from build123d import *

# Parameters (mm, degrees)
F0_W      = 12.7
F0_H      = 114.3
F1_DEPTH  = 12.7
F2_W      = 6.35
F2_H      = 12.7
F3_DEPTH  = 12.701
F4_R      = 2.794
F5_DEPTH  = 6.351
F6_R      = 4.7625
F7_DEPTH  = 5.08
F8_R      = 2.413
F9_DEPTH  = 9.525
F10_R     = 2.413
F11_DEPTH = 9.525


with BuildPart() as f1:
    # F0 (on Right) → F1 (new body)
    with BuildSketch(Plane.YZ):
        with Locations((-6.35, 0)):
            Rectangle(F0_W, F0_H)
    extrude(amount=F1_DEPTH)

    # F2 (on face) → F3 (cut, through all)
    with BuildSketch(Plane(origin=(0, 0, 0), x_dir=(-1, 0, 0), z_dir=(0, 1, 0))):
        with Locations((-3.175, 25.4)):
            Rectangle(F2_W, F2_H)
        with Locations((-3.175, -25.4)):
            Rectangle(F2_W, F2_H)
    extrude(amount=-F3_DEPTH, mode=Mode.SUBTRACT)

    # F4 (on face) → F5 (cut, through all)
    with BuildSketch(Plane(origin=(6.35, 0, 0), x_dir=(0, -1, 0), z_dir=(-1, 0, 0))):
        with Locations((6.35, 25.4)):
            Circle(F4_R)
        with Locations((6.35, -25.4)):
            Circle(F4_R)
    extrude(amount=-F5_DEPTH, mode=Mode.SUBTRACT)

    # F6 (on face) → F7 (cut)
    with BuildSketch(Plane.YZ.offset(12.7)):
        with Locations((-6.35, 25.4)):
            Circle(F6_R)
        with Locations((-6.35, -25.4)):
            Circle(F6_R)
    extrude(amount=-F7_DEPTH, mode=Mode.SUBTRACT)

    # F8 (on face) → F9 (cut)
    with BuildSketch(Plane.XY.offset(57.15)):
        with Locations((6.35, -6.35)):
            Circle(F8_R)
    extrude(amount=-F9_DEPTH, mode=Mode.SUBTRACT)

    # F10 (on face) → F11 (cut)
    with BuildSketch(Plane(origin=(0, 0, -57.15), x_dir=(1, 0, 0), z_dir=(0, 0, -1))):
        with Locations((6.35, 6.35)):
            Circle(F10_R)
    extrude(amount=-F11_DEPTH, mode=Mode.SUBTRACT)


solid = f1.part
Work out the finished part from the listing and answer in its coordinate system (mm). A direction names the side the tool comes from. Give positions to 0.01 mm unless a question says otherwise; leave off trailing zeros. Order: outer loops, then holes, each group sorted by start corner. A loop starts at its lowest first (then second) coordinate and runs counter-clockwise, first axis right, second up. Notation, with made-up numbers: (7.25, -23) -> (32.25, -23) arc R23 cw to (32.25, -11) -> close; hole circle Ø2 at (-33.75, 12). An arc over 180 degrees is marked (long way). Answer as a JSON object with one key per item and string values. Group by question number.
1. Section A-A on x = 2 is taken. Determine the outline of the cut face in (y, z), plus the area to 3 significant figures.
2. A tool of negligible diameter and unlimited length cuts with its end or side. For faces 4 (the cylindrical face through (8.652, -7.075, -52.454)), 5 (the cylindrical face through (10.2, -6.97, 30.12)), 6 (the flat face through (3, -6, 31.75)), 7 (the flat face through (6, -6, 47.625)), from which of +Z, -Z, +X, -X, +Y, -Y can it reach the whole face along a straight path? Write none if from no direction.
3. Consider line 1 along Z through (x, y) = (10.25, -6.5); line 2 along Z through (x, y) = (7.1, -6.35) (3 decimals); line 3 along X through (y, z) = (-6.35, -50.5). Determine where each line is inside the solid, lowest interval first. Write a range as [from, to].
4. The mould has two halves that part along Y. Classify faces 1 (the flat face through (6, -6, -47.625)), 2 (the flat face through (0, -6, 0)), 3 (the flat face through (6, 0, -1)): released by +Y, released by -Y, zero draft, split by the parting line, or undercut.
5. Section B-B on z = -25.4 is taken. Determine the outline of the cut face in (x, y), plus the area to 3 significant figures.
6. Section C-C on x = 11.25 is taken. Count the separate pieces of the cut face and the enclosed holes in it, plus the area to 3 significant figures.
7. Flat-ended cylindrical pins translate along their axes: pin 1 Ø5 at (y, z) = (-4.5, -24.5) entering from +X; pin 2 Ø2 at (y, z) = (-3, 24) entering from -X; pin 3 Ø4.5 at (x, y) = (6.35, -6.35) entering from +Z (3 decimals). Find the tip coordinate at first contact, or state that the pin passes through.
Result sheet:
{
 "1": {"outline": "(-12.7, -57.15) -> (0, -57.15) -> (0, -31.75) -> (-12.7, -31.75) -> close; (-12.7, -19.05) -> (0, -19.05) -> (0, 19.05) -> (-12.7, 19.05) -> close; (-12.7, 31.75) -> (0, 31.75) -> (0, 57.15) -> (-12.7, 57.15) -> close", "area": "1,130 mm^2"},
 "2": {"face 4": "-Z", "face 5": "+X", "face 6": "-X, +Y, -Y", "face 7": "+Z"},
 "3": {"line 1": "z = [-57.15, -30.16], [-20.64, 20.64], [30.16, 57.15]", "line 2": "z = [-47.625, -28.194], [-22.606, 22.606], [28.194, 47.625]", "line 3": "x = [0, 3.94], [8.76, 12.7]"},
 "4": {"face 1": "undercut", "face 2": "zero draft", "face 3": "released by +Y"},
 "5": {"outline": "(6.35, -12.7) -> (12.7, -12.7) -> (12.7, -11.11) -> (7.62, -11.11) -> (7.62, -9.14) -> (6.35, -9.14) -> close; (6.35, -3.56) -> (7.62, -3.56) -> (7.62, -1.59) -> (12.7, -1.59) -> (12.7, 0) -> (6.35, 0) -> close", "area": "25.2 mm^2"},
 "6": {"separate pieces": "1", "enclosed holes": "2", "area": "1,310 mm^2"},
 "7": {"pin 1": "stops at x = 7.62", "pin 2": "stops at x = 6.35", "pin 3": "stops at z = 47.625"}
}
